from build123d import *
from build123d.topology import SkipClean

# Parameters (mm, degrees)
SKETCH_2_W          = 168
SKETCH_2_H          = 190
EXTRUDE_1_DEPTH     = 35
CUT_EXTRUDE_1_REACH = 133.552
SKETCH_3_R          = 3.75
CUT_EXTRUDE_2_REACH = 133.552
SKETCH_4_R          = 4
SKETCH_5_R          = 20
CUT_EXTRUDE_3_DEPTH = 3
FILLET_1_R          = 25
EXTRUDE_2_DEPTH     = 300
CUT_EXTRUDE_START   = 260
CUT_EXTRUDE_4_DEPTH = 260
EXTRUDE_3_DEPTH     = 7.5
SKETCH_12_R         = 4.25
CUT_EXTRUDE_5_DEPTH = 366.418937659


with BuildPart() as part:
    # Sketch 2 → Extrude 1 (new body)
    with BuildSketch(Plane(origin=(0, 0, 0), x_dir=(1, 0, 0), z_dir=(0, 1, 0))):
        Rectangle(SKETCH_2_W, SKETCH_2_H)
    extrude(amount=EXTRUDE_1_DEPTH)

    # Sketch 3 → Cut-Extrude 1 (cut, up to next)
    with BuildSketch(Plane(origin=(0, 35, 0), x_dir=(1, 0, 0), z_dir=(0, 1, 0)), mode=Mode.PRIVATE) as cut_extrude_1_sk1:
        with Locations(Location((0, 75, 0), (0, 0, 270))):
            Circle(SKETCH_3_R)
    cut_extrude_1_tool1 = extrude(cut_extrude_1_sk1.sketch, amount=-CUT_EXTRUDE_1_REACH, mode=Mode.PRIVATE) & part.part
    # Sketch 3 → Cut-Extrude 1 (cut, up to next)
    with BuildSketch(Plane(origin=(0, 35, 0), x_dir=(1, 0, 0), z_dir=(0, 1, 0)), mode=Mode.PRIVATE) as cut_extrude_1_sk2:
        with Locations(Location((0, -75, 0), (0, 0, 270))):
            Circle(SKETCH_3_R)
    cut_extrude_1_tool2 = extrude(cut_extrude_1_sk2.sketch, amount=-CUT_EXTRUDE_1_REACH, mode=Mode.PRIVATE) & part.part
    add(cut_extrude_1_tool1.solids().sort_by_distance((0, 35, -75))[0], mode=Mode.SUBTRACT)
    add(cut_extrude_1_tool2.solids().sort_by_distance((0, 35, 75))[0], mode=Mode.SUBTRACT)

    # Sketch 4 → Cut-Extrude 2 (cut, up to next)
    with BuildSketch(Plane(origin=(0, 35, 0), x_dir=(1, 0, 0), z_dir=(0, 1, 0)), mode=Mode.PRIVATE) as cut_extrude_2_sk1:
        with Locations(Location((-50, 65, 0), (0, 0, 270))):
            Circle(SKETCH_4_R)
    cut_extrude_2_tool1 = extrude(cut_extrude_2_sk1.sketch, amount=-CUT_EXTRUDE_2_REACH, mode=Mode.PRIVATE) & part.part
    # Sketch 4 → Cut-Extrude 2 (cut, up to next)
    with BuildSketch(Plane(origin=(0, 35, 0), x_dir=(1, 0, 0), z_dir=(0, 1, 0)), mode=Mode.PRIVATE) as cut_extrude_2_sk2:
        with Locations(Location((50, 65, 0), (0, 0, 270))):
            Circle(SKETCH_4_R)
    cut_extrude_2_tool2 = extrude(cut_extrude_2_sk2.sketch, amount=-CUT_EXTRUDE_2_REACH, mode=Mode.PRIVATE) & part.part
    # Sketch 4 → Cut-Extrude 2 (cut, up to next)
    with BuildSketch(Plane(origin=(0, 35, 0), x_dir=(1, 0, 0), z_dir=(0, 1, 0)), mode=Mode.PRIVATE) as cut_extrude_2_sk3:
        with Locations(Location((-50, -65, 0), (0, 0, 270))):
            Circle(SKETCH_4_R)
    cut_extrude_2_tool3 = extrude(cut_extrude_2_sk3.sketch, amount=-CUT_EXTRUDE_2_REACH, mode=Mode.PRIVATE) & part.part
    # Sketch 4 → Cut-Extrude 2 (cut, up to next)
    with BuildSketch(Plane(origin=(0, 35, 0), x_dir=(1, 0, 0), z_dir=(0, 1, 0)), mode=Mode.PRIVATE) as cut_extrude_2_sk4:
        with Locations(Location((50, -65, 0), (0, 0, 270))):
            Circle(SKETCH_4_R)
    cut_extrude_2_tool4 = extrude(cut_extrude_2_sk4.sketch, amount=-CUT_EXTRUDE_2_REACH, mode=Mode.PRIVATE) & part.part
    add(cut_extrude_2_tool1.solids().sort_by_distance((-50, 35, -65))[0], mode=Mode.SUBTRACT)
    add(cut_extrude_2_tool2.solids().sort_by_distance((50, 35, -65))[0], mode=Mode.SUBTRACT)
    add(cut_extrude_2_tool3.solids().sort_by_distance((-50, 35, 65))[0], mode=Mode.SUBTRACT)
    add(cut_extrude_2_tool4.solids().sort_by_distance((50, 35, 65))[0], mode=Mode.SUBTRACT)

    # Sketch 5 → Cut-Extrude 3 (cut)
    with BuildSketch(Plane(origin=(0, 35, 0), x_dir=(1, 0, 0), z_dir=(0, 1, 0))):
        with Locations(Location((-50, 65, 0), (0, 0, 270))):
            Circle(SKETCH_5_R)
        with Locations(Location((50, 65, 0), (0, 0, 270))):
            Circle(SKETCH_5_R)
        with Locations(Location((50, -65, 0), (0, 0, 270))):
            Circle(SKETCH_5_R)
        with Locations(Location((-50, -65, 0), (0, 0, 270))):
            Circle(SKETCH_5_R)
    extrude(amount=-CUT_EXTRUDE_3_DEPTH, mode=Mode.SUBTRACT)

    # Fillet 1
    fillet_1_edges = [part.edges().sort_by_distance(p)[0] for p in [
        (-84, 17.5, -95),
        (84, 17.5, -95),
        (84, 17.5, 95),
        (-84, 17.5, 95),
    ]]
    fillet(fillet_1_edges, radius=FILLET_1_R)

    # Sketch 8 → Extrude 2 (add)
    with BuildSketch(Plane(origin=(0, 315, 0), x_dir=(1, 0, 0), z_dir=(0, 1, 0))):
        with BuildLine():
            Line((-109, 16), (-109, -16))
            Line((-109, -16), (-159, -16))
            Line((-159, -16), (-159, -35))
            ThreePointArc((-159, -35), (-157.535533906, -38.535533906), (-154, -40))
            Line((-154, -40), (-143.874685928, -40))
            ThreePointArc((-143.874685928, -40), (-137.166481995, -42.583801513), (-133.924811557, -49))
            ThreePointArc((-133.924811557, -49), (-121.126812284, -62.348456806), (-105.096341116, -53.129233486))
            ThreePointArc((-105.096341116, -53.129233486), (-98.786961451, -45.541087589), (-89.248249261, -43.01102837))
            ThreePointArc((-89.248249261, -43.01102837), (-85.553352811, -41.639435016), (-84, -38.017194942))
            Line((-84, -38.017194942), (-84, 38.017194942))
            ThreePointArc((-84, 38.017194942), (-85.553352811, 41.639435016), (-89.248249261, 43.01102837))
            ThreePointArc((-89.248249261, 43.01102837), (-98.786961451, 45.541087589), (-105.096341116, 53.129233486))
            ThreePointArc((-105.096341116, 53.129233486), (-121.126812284, 62.348456806), (-133.924811557, 49))
            ThreePointArc((-133.924811557, 49), (-137.166481995, 42.583801513), (-143.874685928, 40))
            Line((-143.874685928, 40), (-154, 40))
            ThreePointArc((-154, 40), (-157.535533906, 38.535533906), (-159, 35))
            Line((-159, 35), (-159, 16))
            Line((-159, 16), (-109, 16))
        make_face()
    extrude(amount=-EXTRUDE_2_DEPTH)

    # Sketch 10 → Cut-Extrude 4 (cut)
    with SkipClean():  # the faces are left unmerged after this step: merging them gives an invalid solid
        with BuildSketch(Plane(origin=(0, 35, 0), x_dir=(1, 0, 0), z_dir=(0, 1, 0)).offset(CUT_EXTRUDE_START)):
            with BuildLine():
                ThreePointArc((-94, 40), (-90.464466094, 38.535533906), (-89, 35))
                Line((-89, 35), (-89, -35))
                ThreePointArc((-89, -35), (-90.464466094, -38.535533906), (-94, -40))
                Line((-94, -40), (-154, -40))
                ThreePointArc((-154, -40), (-157.535533906, -38.535533906), (-159, -35))
                Line((-159, -35), (-159, -16))
                Line((-159, -16), (-166.391829747, -16))
                Line((-166.391829747, -16), (-166.391829747, -67.593352797))
                Line((-166.391829747, -67.593352797), (-78.896973025, -67.593352797))
                Line((-78.896973025, -67.593352797), (-78.896973025, 67.593352797))
                Line((-78.896973025, 67.593352797), (-166.391829747, 67.593352797))
                Line((-166.391829747, 67.593352797), (-166.391829747, 16))
                Line((-166.391829747, 16), (-159, 16))
                Line((-159, 16), (-159, 35))
                ThreePointArc((-159, 35), (-157.535533906, 38.535533906), (-154, 40))
                Line((-154, 40), (-94, 40))
            make_face()
        extrude(amount=-CUT_EXTRUDE_4_DEPTH, mode=Mode.SUBTRACT)
    add(part.part.scale(1), mode=Mode.REPLACE)  # the faces are merged on a copy

    # Sketch 11 → Extrude 3 (add, symmetric)
    with BuildSketch(Plane.XY):
        Polygon((-84, 295), (71.5, 35), (-89.248249261, 35), (-89.248249261, 295), align=None)
    extrude(amount=EXTRUDE_3_DEPTH, both=True)

    # Sketch 12 → Cut-Extrude 5 (cut, through all)
    with BuildSketch(Plane(origin=(0, 315, 0), x_dir=(1, 0, 0), z_dir=(0, 1, 0))):
        with Locations(Location((-119, 47.5, 0), (0, 0, 270))):
            Circle(SKETCH_12_R)
        with Locations(Location((-119, -47.5, 0), (0, 0, 270))):
            Circle(SKETCH_12_R)
    extrude(amount=-CUT_EXTRUDE_5_DEPTH, mode=Mode.SUBTRACT)


solid = part.part
The listing builds one solid part. Answer for the finished solid, in the listing's coordinates (mm). A direction names the side the tool comes from. Coordinates: 2 decimals unless noted, no trailing zeros. Order: outer loops, then holes, each group sorted by start corner. A loop starts at its lowest first (then second) coordinate and runs counter-clockwise, first axis right, second up.
Q1. Given P1, Ø6, axis at x = 0, z = -75, coming from the +Y side; P2, Ø15, axis at x = -137.5, y = 118.5, coming from the +Z side; P3, Ø3, axis at x = -44, y = 98.5, coming from the -Z side; P4, Ø2, axis at x = -4, z = -5.5, coming from the +Y side, each flat-ended and moving along its own axis, determine where each tip first touches the part or whether it passes through.
Q2. Consider line 1 (X direction, y = 10, z = 65); line 2 (X direction, y = 33.35, z = 65); line 3 (Z direction, x = -125, y = 278.5). Determine where each line is inside the solid, lowest interval first.
Q3. A cutting plane is placed at D-D, the plane z = 75. Write down the section's boundary in (x, y), and give its area (3 significant figures).
Q4. A cutting plane is placed at A-A, the plane x = -119. State how many separate pieces and enclosed holes the cut face has, and give its area (3 significant figures).
Q5. A cutting plane is placed at B-B, the plane z = 2.5. Write down the section's boundary in (x, y).
Q6. Which of the six approach directions +Z, -Z, +X, -X, +Y, -Y give full straight-line access (tool end or side, diameter ignored) to faces 1 (the face through (-43.993, 33.521, 84.076)), 2 (the face through (-159, 167, -26))?
Q7. A cutting plane is placed at C-C, the plane y = 243. Write down the section's boundary in (x, z), and give its area (3 significant figures).
Q8. For a pull along Z with two mould halves and no side action, classify faces 3 (the face through (-105, 315, -1)), 4 (the face through (-98.905, 25.14, 45.617)), 5 (the face through (-49.7, 32, 69.2)), 6 (the face through (-51.532, 16.224, 68.695)) as pulls with the +Z half, pulls with the -Z half, needs draft (parallel to the pull), parting line crosses it, or undercut.
Answers follow:
1. P1: passes through
1. P2: stops at z = 40
1. P3: stops at z = -7.5
1. P4: stops at y = 162.91
2. line 1: x = -84 to -54, -46 to 46, 54 to 84
2. line 2: x = -84 to -70, -30 to 30, 70 to 84
2. line 3: z = -40 to -16, 16 to 40
3. outline: (-83.49, 0) - (-3.75, 0) - (-3.75, 35) - (-32.68, 35) - (-32.68, 32) - (-67.32, 32) - (-67.32, 35) - (-83.49, 35) - close; (3.75, 0) - (83.49, 0) - (83.49, 35) - (67.32, 35) - (67.32, 32) - (32.68, 32) - (32.68, 35) - (3.75, 35) - close
3. area: 5,370 mm2
4. separate pieces: 6
4. enclosed holes: 0
4. area: 15,500 mm2
5. outline: (-109, 15) - (-84, 15) - (-84, 0) - (84, 0) - (84, 35) - (71.5, 35) - (-84, 295) - (-84, 315) - (-109, 315) - close
6. face 1: +Y
6. face 2: +Z, -Z, -X, +Y, -Y
7. outline: (-159, -35) arc R5 ccw to (-154, -40) - (-94, -40) arc R5 ccw to (-89, -35) - (-89, -7.5) - (-52.9, -7.5) - (-52.9, 7.5) - (-89, 7.5) - (-89, 35) arc R5 ccw to (-94, 40) - (-154, 40) arc R5 ccw to (-159, 35) - (-159, 16) - (-109, 16) - (-109, -16) - (-159, -16) - close
7. area: 4,520 mm2
8. face 3: needs draft
8. face 4: pulls with the +Z half
8. face 5: undercut
8. face 6: undercut
